Can you work these out from the model? Positions are in its coordinate system, mm. Face numbers are marked on the shaded views. A direction names the side the tool comes from. Round coordinates to 2 decimals unless told otherwise and drop trailing zeros. Loops run counter-clockwise (first coordinate to the right, second up) from the corner with the lowest first, then second, coordinate; pieces in that order, holes last. Notation, with made-up numbers: (42.5, 87) -> (97.5, 87) arc R8 cw to (97.5, 94) -> close; hole circle Ø8 at (-21, 41). An arc over 180 degrees is marked (long way). Answer as a JSON object with one key per item and string values.
Autodesk Inventor part; units mm, degrees
ref_plane "YZ Plane" through (0, 0, 0) normal (1, 0, 0) x (0, 1, 0)
ref_plane "XZ Plane" through (0, 0, 0) normal (0, 1, 0) x (-1, 0, 0)
ref_plane "XY Plane" through (0, 0, 0) normal (0, 0, 1) x (1, 0, 0)
sketch "スケッチ1" plane through (0, 0, 0) normal (1, 0, 0) x (0, 1, 0)
  line L0 (60, -16.042) -> (-60, -16.042)
  line L1 (-60, -16.042) -> (-60, 16.042)
  line L2 (-60, 16.042) -> (60, 16.042)
  line L3 (60, 16.042) -> (60, -16.042)
  line L4 (60, -16.042) -> (-60, 16.042) construction
  line L5 (-60, -16.042) -> (60, 16.042) construction
  line L6 (-56, 13.625) -> (56, 13.625)
  line L7 (56, 13.625) -> (56, 10.625)
  line L8 (56, 10.625) -> (-56, 10.625)
  line L9 (-56, 10.625) -> (-56, 13.625)
  line L10 (-56, -10.625) -> (56, -10.625)
  line L11 (56, -10.625) -> (56, -13.625)
  line L12 (56, -13.625) -> (-56, -13.625)
  line L13 (-56, -13.625) -> (-56, -10.625)
  line L14 (60, -16.042) -> (-60, -16.042)
  line L15 (-60, -16.042) -> (-60, -29.5)
  line L16 (-60, -29.5) -> (60, -29.5)
  line L17 (60, -29.5) -> (60, -16.042)
  line L18 (-60, 16.042) -> (60, 16.042)
  line L19 (60, 16.042) -> (60, 24.5)
  line L20 (60, 24.5) -> (-60, 24.5)
  line L21 (-60, 24.5) -> (-60, 16.042)
  line L22 (15, 24.5) -> (-15, 24.5)
  line L23 (-15, 24.5) -> (-15, 39.5)
  line L24 (-15, 39.5) -> (15, 39.5)
  line L25 (15, 39.5) -> (15, 24.5)
  line L26 (20, -29.5) -> (10, -29.5)
  line L27 (-10, -29.5) -> (-20, -29.5)
  circle A0 centre (9, 33.5) radius 1.6
  circle A1 centre (-9, 33.5) radius 1.6
  line L28 (60, 0) -> (-60, 0)
  line L29 (15, -29.5) -> (-15, -29.5)
  line L30 (-15, -29.5) -> (-15, -44.5)
  line L31 (-15, -44.5) -> (15, -44.5)
  line L32 (15, -44.5) -> (15, -29.5)
  circle A2 centre (-9, -38.5) radius 1.6
  circle A3 centre (9, -38.5) radius 1.6
  point P0 (0, 0)
  point P1 (0, 0)
  point P2 (56, 12.125)
  point P3 (56, -12.125)
  point P4 (0, 0)
  point P5 (-15, 24.5)
  point P6 (-15, -29.5)
  dimension "d1" = 120
  dimension "d3" = 12.125
  dimension "d6" = 3
  dimension "d11" = 12.125
  dimension "d15" = 2.417
  dimension "d26" = 4
  dimension "d27" = 4
  dimension "d41" = 29.5
  dimension "d53" = 54
  dimension "d72" = 15
  dimension "d74" = 15
  dimension "d75" = 30
  dimension "d79" = 6
  dimension "d80" = 3.2
  dimension "d92" = 18
  dimension "d97" = 15
  dimension "d101" = 72
  dimension "d106" = 9
extrude "押し出し1" add sketch "スケッチ1" along normal blind 2
sketch "スケッチ3" plane through (0, 0, 0) normal (-1, 0, 0) x (0, 0, 1)
  line L0 (-29.5, 60) -> (24.5, 60)
  line L1 (5.575, 60) -> (4.575, 60)
  line L2 (4.575, 60) -> (4.575, 7)
  line L3 (4.575, 7) -> (5.575, 7)
  line L4 (5.575, 7) -> (5.575, 60)
  line L5 (16.675, 60) -> (15.675, 60)
  line L6 (15.675, 60) -> (15.675, 0)
  line L7 (15.675, 0) -> (16.675, 0)
  line L8 (16.675, 0) -> (16.675, 60)
  line L9 (0, 0) -> (4.575, 0)
  line L10 (0, 0) -> (0, 19.0491)
  line L11 (5.575, -60) -> (4.575, -60)
  line L12 (4.575, -60) -> (4.575, -7)
  line L13 (4.575, -7) -> (5.575, -7)
  line L14 (5.575, -7) -> (5.575, -60)
  line L15 (16.675, -60) -> (15.675, -60)
  line L16 (15.675, -60) -> (15.675, 0)
  line L17 (16.675, 0) -> (16.675, -60)
  line L18 (-5.575, 60) -> (-4.575, 60)
  line L19 (-4.575, 60) -> (-4.575, 7)
  line L20 (-4.575, 7) -> (-5.575, 7)
  line L21 (-5.575, 7) -> (-5.575, 60)
  line L22 (-16.675, 60) -> (-15.675, 60)
  line L23 (-15.675, 60) -> (-15.675, 0)
  line L24 (-15.675, 0) -> (-16.675, 0)
  line L25 (-16.675, 0) -> (-16.675, 60)
  line L26 (-5.575, -60) -> (-4.575, -60)
  line L27 (-4.575, -60) -> (-4.575, -7)
  line L28 (-4.575, -7) -> (-5.575, -7)
  line L29 (-5.575, -7) -> (-5.575, -60)
  line L30 (-16.675, -60) -> (-15.675, -60)
  line L31 (-15.675, -60) -> (-15.675, 0)
  line L32 (-16.675, 0) -> (-16.675, -60)
  line L33 (5.575, 60) -> (15.675, 60)
  line L34 (15.675, 60) -> (15.675, 59)
  line L35 (15.675, 59) -> (5.575, 59)
  line L36 (5.575, 59) -> (5.575, 60)
  line L37 (-5.575, -60) -> (-15.675, -60)
  line L38 (-15.675, -60) -> (-15.675, -59)
  line L39 (-15.675, -59) -> (-5.575, -59)
  line L40 (-5.575, -59) -> (-5.575, -60)
  point P0 (-15.675, 60)
  point P1 (-16.675, 60)
  point P2 (15.675, 60)
  point P3 (0, 9.5245)
  point P4 (-5.575, -59)
  point P5 (5.575, 59)
  dimension "d31" = 1
  dimension "d33" = 1
  dimension "d34" = 60
  dimension "d35" = 10.1
  dimension "d36" = 7
  dimension "d61" = 5.575
  dimension "d62" = 1
  dimension "d63" = 1
extrude "押し出し4" add sketch "スケッチ3" along normal blind 4
equation "\"d2\" = 0.25 * d0"
equation "\"d73\" = d72"
equation "\"d78\" = 0.5 * d72"
properties part number "hand_box1"
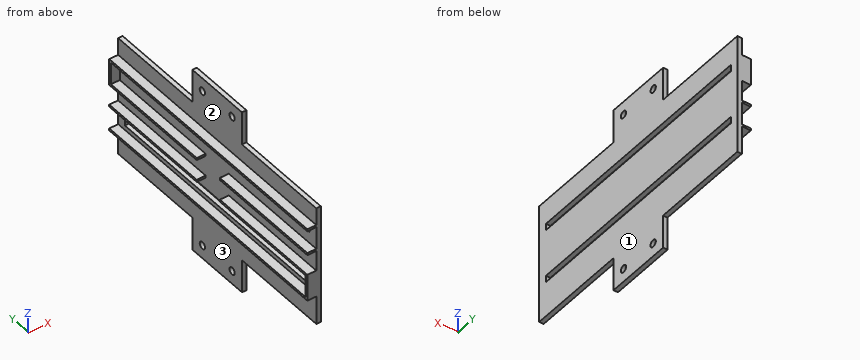
Q1. I want a section at D-D, the plane y = -9. Give the number of separate pieces and of enclosed holes in the cut face, then the cut area to 3 significant figures.
Determined:
{"separate pieces": "5", "enclosed holes": "0", "area": "159 mm²"}
Q2. On a 3-axis mill with a long thin cutter (end or side, diameter ignored), from which of +Z, -Z, +X, -X, +Y, -Y can I reach the whole of each face in a straight line? I mean the marked faces 1, 2 and 3. Say none if no direction works.
Determined:
{"face 1": "+Z, -Z, +X, +Y, -Y", "face 2": "+Z, -X, +Y, -Y", "face 3": "-Z, -X, +Y, -Y"}
Q3. I want a section at A-A, the plane y = -33. Write out the boundary of the cut face in (x, z) (3 decimals), then the cut area to 3 significant figures.
Determined:
{"outline": "(-4, -16.675) -> (0, -16.675) -> (0, -29.5) -> (2, -29.5) -> (2, -13.625) -> (0, -13.625) -> (0, -15.675) -> (-4, -15.675) -> close; (-4, -5.575) -> (0, -5.575) -> (0, -10.625) -> (2, -10.625) -> (2, 10.625) -> (0, 10.625) -> (0, 5.575) -> (-4, 5.575) -> (-4, 4.575) -> (0, 4.575) -> (0, -4.575) -> (-4, -4.575) -> close; (-4, 15.675) -> (0, 15.675) -> (0, 13.625) -> (2, 13.625) -> (2, 24.5) -> (0, 24.5) -> (0, 16.675) -> (-4, 16.675) -> close", "area": "112 mm²"}
Q4. I'm going to push flat-ended pins straight in: pin 1 (0.6 mm diameter, centred on x = 1, z = -34.5, fed in from +Y); pin 2 (9.5 mm diameter, centred on y = 11.5, z = -4, fed in from -X); pin 3 (7 mm diameter, centred on y = 0.5, z = 28.5, fed in from -X); pin 4 (1 mm diameter, centred on x = 1, y = 21, fed in from -Z). Where does each tip first touch, or does it pass through?
Determined:
{"pin 1": "y = 15", "pin 2": "x = -4", "pin 3": "x = 0", "pin 4": "z = -29.5"}
Q5. If I drill on L1, parallel to Z at x = -2.4, y = 54.5 (3 decimals); L2, parallel to Z at x = 0.65, y = -9 (3 decimals); L3, parallel to Z at x = 1.2, y = -47 (3 decimals), over which ranges is the centre line in solid material (lowest first)? Write a range as [from, to].
Determined:
{"L1": "[-16.675, -15.675], [-5.575, -4.575], [4.575, 5.575], [15.675, 16.675]", "L2": "[-44.5, -40.1], [-36.9, -13.625], [-10.625, 10.625], [13.625, 31.9], [35.1, 39.5]", "L3": "[-29.5, -13.625], [-10.625, 10.625], [13.625, 24.5]"}
Q6. I want a section at C-C, the plane x = -1.7. Write out the boundary of the cut face in (y, z) (3 decimals), then the cut area to 3 significant figures.
Determined:
{"outline": "(-60, -16.675) -> (60, -16.675) -> (60, -15.675) -> (-59, -15.675) -> (-59, -5.575) -> (-7, -5.575) -> (-7, -4.575) -> (-60, -4.575) -> close; (-60, 4.575) -> (-7, 4.575) -> (-7, 5.575) -> (-60, 5.575) -> close; (-60, 15.675) -> (59, 15.675) -> (59, 5.575) -> (7, 5.575) -> (7, 4.575) -> (60, 4.575) -> (60, 16.675) -> (-60, 16.675) -> close; (7, -5.575) -> (60, -5.575) -> (60, -4.575) -> (7, -4.575) -> close", "area": "472 mm²"}
Q7. I want a section at B-B, the plane z = -38.5. Write out the boundary of the cut face in (x, y).
Determined:
{"outline": "(0, -15) -> (2, -15) -> (2, -10.6) -> (0, -10.6) -> close; (0, -7.4) -> (2, -7.4) -> (2, 7.4) -> (0, 7.4) -> close; (0, 10.6) -> (2, 10.6) -> (2, 15) -> (0, 15) -> close"}
